```python
from build123d import *

# Parameters (mm, degrees)
SKETCH_1_W          = 13
SKETCH_1_H          = 20
EXTRUDE_1_DEPTH     = 5
SKETCH_3_W          = 3
SKETCH_3_H          = 20
EXTRUDE_2_DEPTH     = 15.7
SKETCH_4_W          = 2
SKETCH_4_H          = 20
EXTRUDE_3_DEPTH     = 15
SKETCH_5_W          = 12
SKETCH_5_H          = 14
CUT_EXTRUDE_1_DEPTH = 21.7
SKETCH_6_R          = 1.75
CUT_EXTRUDE_2_DEPTH = 6


with BuildPart() as part:
    # 草图1 → 凸台-拉伸1 (new body)
    with BuildSketch(Plane.XY):
        with Locations((6.5, 10)):
            Rectangle(SKETCH_1_W, SKETCH_1_H)
    extrude(amount=EXTRUDE_1_DEPTH)

    # 草图3 → 凸台-拉伸2 (add)
    with BuildSketch(Plane.XY.offset(5)):
        with Locations((11.5, 10)):
            Rectangle(SKETCH_3_W, SKETCH_3_H)
    extrude(amount=EXTRUDE_2_DEPTH)

    # 草图4 → 凸台-拉伸3 (add)
    with BuildSketch(Plane.ZY.offset(-10)):
        with Locations((19.7, 10)):
            Rectangle(SKETCH_4_W, SKETCH_4_H)
    extrude(amount=-EXTRUDE_3_DEPTH)

    # 草图5 → 切除-拉伸1 (cut, through all)
    with BuildSketch(Plane.XY.offset(20.7)):
        with Locations((19, 7)):
            Rectangle(SKETCH_5_W, SKETCH_5_H)
    extrude(amount=-CUT_EXTRUDE_1_DEPTH, mode=Mode.SUBTRACT)

    # 草图6 → 切除-拉伸2 (cut, through all)
    with BuildSketch(Plane.XY.offset(5)):
        with Locations((5, 15)):
            Circle(SKETCH_6_R)
        with Locations((5, 5)):
            Circle(SKETCH_6_R)
    extrude(amount=-CUT_EXTRUDE_2_DEPTH, mode=Mode.SUBTRACT)


solid = part.part
```
Geometry check sheet. Reference: the model listing, model coordinates, mm. A direction names the side the tool comes from. Coordinates: 2 decimals unless noted, no trailing zeros. Order: outer loops, then holes, each group sorted by start corner. A loop starts at its lowest first (then second) coordinate and runs counter-clockwise, first axis right, second up.
Q1. Depth check by flat-ended pin: pin 1 Ø1.6 at (x, z) = (18.5, 19.5) entering from -Y; pin 2 Ø5 at (y, z) = (10, 9.5) entering from +X; pin 3 Ø4 at (y, z) = (7, 14) entering from -X. Enter the tip coordinate at first touch or a pass-through.
Reply:
pin 1: stops at y = 14
pin 2: stops at x = 13
pin 3: stops at x = 10
Q2. Tool access check on faces 5 (the face through (19, 17, 18.7)), 6 (the face through (10, 10, 13)), 7 (the face through (25, 17, 20)), 8 (the face through (19, 14, 20)). Record the directions out of +Z, -Z, +X, -X, +Y, -Y that give a thin tool (end or side, any length) a straight path to the whole face; none if there is none.
Reply:
face 5: -Z, +X, +Y, -Y
face 6: +Z, -X, +Y, -Y
face 7: +Z, -Z, +X, +Y, -Y
face 8: +Z, -Z, +X, -Y
Q3. Thickness scan on probe 1 along Y at (x, z) = (5, 2.1); probe 2 along X at (y, z) = (13.75, 13.5); probe 3 along Z at (x, y) = (8, 7.25). Record the ranges inside material, lowest first.
Reply:
probe 1: y = 0 to 3.25, 6.75 to 13.25, 16.75 to 20
probe 2: x = 10 to 13
probe 3: z = 0 to 5
Q4. Sectioned sample at D-D on z = 2.75. Record the cut outline in (x, y).
Reply:
outline: (0, 0) - (13, 0) - (13, 20) - (0, 20) - close; hole circle Ø3.5 at (5, 5); hole circle Ø3.5 at (5, 15)
Q5. Draft check along Y on faces 1 (the face through (16, 15, 20.7)), 2 (the face through (11, 20, 9)), 3 (the face through (4.772, 16.735, 2.535)), 4 (the face through (3.61, 3.94, 2.54)). Enter one of: released by +Y, released by -Y, zero draft, split by the parting line, or undercut.
Reply:
face 1: zero draft
face 2: released by +Y
face 3: undercut
face 4: undercut
Q6. Sectioned sample at A-A on x = 5. Record the cut outline in (y, z).
Reply:
outline: (0, 0) - (3.25, 0) - (3.25, 5) - (0, 5) - close; (6.75, 0) - (13.25, 0) - (13.25, 5) - (6.75, 5) - close; (16.75, 0) - (20, 0) - (20, 5) - (16.75, 5) - close
Q7. Sectioned sample at C-C on y = 17.5. Record the cut outline in (x, z).
Reply:
outline: (0, 0) - (13, 0) - (13, 18.7) - (25, 18.7) - (25, 20.7) - (10, 20.7) - (10, 5) - (0, 5) - close
Q8. Sectioned sample at B-B on y = 15. Record the cut outline in (x, z), and give its area (3 significant figures).
Reply:
outline: (0, 0) - (3.25, 0) - (3.25, 5) - (0, 5) - close; (6.75, 0) - (13, 0) - (13, 18.7) - (25, 18.7) - (25, 20.7) - (10, 20.7) - (10, 5) - (6.75, 5) - close
area: 119 mm2
